from build123d import *

# Parameters (mm, degrees)
SKETCH3_R           = 15
BOSS_EXTRUDE1_DEPTH = 25
SKETCH5_W           = 218
SKETCH5_H           = 50
CUT_EXTRUDE1_DEPTH  = 20
SKETCH7_W           = 15
SKETCH7_H           = 50
CUT_EXTRUDE3_DEPTH  = 219
SKETCH8_R           = 15
SKETCH8_R_2         = 10
BOSS_EXTRUDE7_DEPTH = 75
SKETCH9_W           = 10
SKETCH9_H           = 50
BOSS_EXTRUDE8_DEPTH = 400
SKETCH10_W          = 40
SKETCH10_H          = 30
SKETCH10_W_2        = 34
SKETCH10_H_2        = 24
BOSS_EXTRUDE9_DEPTH = 400


with BuildPart() as part:
    # Sketch3 → Boss-Extrude1 (new body)
    with BuildSketch(Plane.XY):
        with BuildLine():
            Line((-68.346942832, 96), (-86.545454545, 46))
            Line((-86.545454545, 46), (-86.545454545, -14))
            Line((-86.545454545, -14), (131.454545455, -14))
            Line((131.454545455, -14), (131.454545455, 96))
            Line((131.454545455, 96), (107.496522982, 96))
            Line((107.496522982, 96), (98.489850442, 70.226827292))
            ThreePointArc((98.489850442, 70.226827292), (81.969545455, 58.5), (65.449240467, 70.226827292))
            Line((65.449240467, 70.226827292), (56.442567927, 96))
            Line((56.442567927, 96), (43.395745829, 96))
            Line((43.395745829, 96), (6.961681078, 61.857864376))
            ThreePointArc((6.961681078, 61.857864376), (-7.180454545, 56), (-21.322590169, 61.857864376))
            Line((-21.322590169, 61.857864376), (-57.753891674, 96))
            Line((-57.753891674, 96), (-68.346942832, 96))
        make_face()
        with Locations((-51.545454545, 15)):
            Circle(SKETCH3_R, mode=Mode.SUBTRACT)
    extrude(amount=BOSS_EXTRUDE1_DEPTH)

    # Sketch5 → Cut-Extrude1 (cut)
    with BuildSketch(Plane.XY.offset(25)):
        with Locations((22.454545455, 71)):
            Rectangle(SKETCH5_W, SKETCH5_H)
    extrude(amount=-CUT_EXTRUDE1_DEPTH, mode=Mode.SUBTRACT)

    # Sketch7 → Cut-Extrude3 (cut, through all)
    with BuildSketch(Plane.ZY.offset(86.545454545)):
        with Locations((12.5, 16)):
            Rectangle(SKETCH7_W, SKETCH7_H)
    extrude(amount=-CUT_EXTRUDE3_DEPTH, mode=Mode.SUBTRACT)

    # Sketch8 → Boss-Extrude7 (add)
    with BuildSketch(Plane(origin=(0, 0, 0), x_dir=(-1, 0, 0), z_dir=(0, 0, -1))):
        with Locations((51.545454545, 15)):
            Circle(SKETCH8_R)
        with Locations((51.545454545, 15)):
            Circle(SKETCH8_R_2, mode=Mode.SUBTRACT)
    extrude(amount=-BOSS_EXTRUDE7_DEPTH)

    # Sketch9 → Boss-Extrude8 (add)
    with BuildSketch(Plane(origin=(0, 0, 0), x_dir=(-1, 0, 0), z_dir=(0, 0, -1))):
        with Locations((81.545454545, 11)):
            Rectangle(SKETCH9_W, SKETCH9_H)
    extrude(amount=BOSS_EXTRUDE8_DEPTH)

    # Sketch10 → Boss-Extrude9 (add)
    with BuildSketch(Plane(origin=(0, 0, 0), x_dir=(-1, 0, 0), z_dir=(0, 0, -1))):
        with Locations((-96.454545455, 21)):
            Rectangle(SKETCH10_W, SKETCH10_H)
        with Locations((-96.454545455, 21)):
            Rectangle(SKETCH10_W_2, SKETCH10_H_2, mode=Mode.SUBTRACT)
    extrude(amount=BOSS_EXTRUDE9_DEPTH)

    # Mirror1: part across plane


with BuildPart() as part_1:
    add(part.part)
    add(part.part.mirror(Plane(origin=(0, 0, -400), x_dir=(1, 0, 0), z_dir=(0, 0, -1))))


solid = part_1.part
Geometry check sheet. Reference: the model listing, model coordinates, mm. A direction names the side the tool comes from. Round coordinates to 2 decimals unless told otherwise and drop trailing zeros. Write each loop counter-clockwise with the first axis right and the second up, starting at its lowest first coordinate (ties: lowest second). Pieces come first, ordered by that corner, then holes.
Item 1: Mould release check, pull along Y, two halves, no side actions. Record for faces 1 (the face through (21, 16, -805)), 2 (the face through (-82, -14, -402)), 3 (the face through (131.455, 29, 4)): +Y half, -Y half, draft (parallel to the pull), parting line (faces both ways), or undercut.
Determined:
face 1: undercut
face 2: -Y half
face 3: draft
Item 2: Go/stop test with flat-tipped pins: pin 1 Ø10 at (x, z) = (24.5, -810.5) entering from +Y; pin 2 Ø17 at (x, z) = (89.5, -488.5) entering from -Y; pin 3 Ø12 at (x, z) = (20, 9.5) entering from +Y. Record where each tip stops, or that it passes through.
Determined:
pin 1: stops at y = 46
pin 2: stops at y = 6
pin 3: stops at y = 77.79
Item 3: Section check B-B (x = 24.5). Record the boundary of the cut face in (y, z), plus the area to 3 significant figures.
Determined:
outline: (-14, -825) - (46, -825) - (46, -805) - (78.29, -805) - (78.29, -800) - (-14, -800) - close; (-14, 0) - (78.29, 0) - (78.29, 5) - (46, 5) - (46, 25) - (-14, 25) - close; hole (-9, -820) - (41, -820) - (41, -805) - (-9, -805) - close; hole (-9, 5) - (41, 5) - (41, 20) - (-9, 20) - close
area: 1,820 mm2
Item 4: Section check A-A (z = -625). Record the boundary of the cut face in (x, y), plus the area to 3 significant figures.
Determined:
outline: (-86.55, -14) - (-76.55, -14) - (-76.55, 36) - (-86.55, 36) - close; (76.45, 6) - (116.45, 6) - (116.45, 36) - (76.45, 36) - close; hole (79.45, 9) - (113.45, 9) - (113.45, 33) - (79.45, 33) - close
area: 884 mm2
Item 5: Access from +Z, -Z, +X, -X, +Y, -Y to the whole of each face (thin tool, end or side, straight path). Record for faces 4 (the face through (-65.4, 9.25, 49.65)), 5 (the face through (97, 36, -406)), 6 (the face through (97, 6, -406)).
Determined:
face 4: +Z
face 5: +X, -X, +Y
face 6: +X, -Y
Item 6: Material ranges on line 1 along Z through (x, y) = (119.5, 40.5); line 2 along Y through (x, z) = (94, -162.5); line 3 along Z through (x, y) = (23, 51), recorded low to high.
Determined:
line 1: z = -825 to -820, -805 to -800, 0 to 5, 20 to 25
line 2: y = 6 to 9, 33 to 36
line 3: z = -805 to -800, 0 to 5
